from build123d import *

# Parameters (mm, degrees)
SKETCH_1_W      = 15
SKETCH_1_H      = 11
SKETCH_1_R      = 1.5
EXTRUDE_1_DEPTH = 1.5
SKETCH_2_W      = 5
SKETCH_2_H      = 5
EXTRUDE_2_DEPTH = 1


with BuildPart() as part:
    # 草图1 → 凸台-拉伸1 (new body)
    with BuildSketch(Plane.XY):
        Rectangle(SKETCH_1_W, SKETCH_1_H)
        with Locations((-5.5, 3.5)):
            Circle(SKETCH_1_R, mode=Mode.SUBTRACT)
        with Locations((5.5, 3.5)):
            Circle(SKETCH_1_R, mode=Mode.SUBTRACT)
    extrude(amount=EXTRUDE_1_DEPTH)

    # 草图2 → 凸台-拉伸2 (add)
    with BuildSketch(Plane.XY.offset(1.5)):
        Rectangle(SKETCH_2_W, SKETCH_2_H)
    extrude(amount=EXTRUDE_2_DEPTH)


solid = part.part
Check sheet for the modelled part. Datum: model origin and axes. Units: mm. A direction names the side the tool comes from. Give positions to 0.01 mm unless a question says otherwise; leave off trailing zeros. Loops run counter-clockwise (first coordinate to the right, second up) from the corner with the lowest first, then second, coordinate; pieces in that order, holes last. Notation, with made-up numbers: M 80.5,-21.75 L 85.5,-21.75 A22 ccw 85.5,-7.75 Z; hole C -36,-14.75 d5. An arc over 180 degrees is marked long. Return JSON: item names as keys, results as strings. Group by question number.
1. Cross-section at D-D on x = 1.25. Record the boundary of the cut face in (y, z).
2. Thickness scan on L1, parallel to Y at x = 5.5, z = 0.7; L2, parallel to Y at x = 1.5, z = 1.95; L3, parallel to X at y = 4.5, z = 0.2. Record the ranges inside material, lowest first.
3. Cross-section at C-C on y = -2.25. Record the boundary of the cut face in (x, z), plus the area to 3 significant figures.
4. Cross-section at A-A on y = 3.5. Record the boundary of the cut face in (x, z), plus the area to 3 significant figures.
5. Mould release check, pull along Y, two halves, no side actions. Record for faces 6 (the cylindrical face through (-7, 3.57, 0.74)), 7 (the flat face through (0, 0, 0)), 8 (the flat face through (0, -5.5, 1)), 9 (the flat face through (0, 5.5, 1)): released by +Y, released by -Y, zero draft, split by the parting line, or undercut.
6. Tool access check on faces 1 (the flat face through (2.5, 0, 2)), 2 (the flat face through (0, 2.5, 2)), 3 (the flat face through (-2.5, 0, 2)), 4 (the flat face through (0, -2.5, 2)), 5 (the flat face through (-7.5, 0, 1)). Record the directions out of +Z, -Z, +X, -X, +Y, -Y that give a thin tool (end or side, any length) a straight path to the whole face; none if there is none.
7. Go/stop test with flat-tipped pins: pin 1 (2.5 mm diameter, centred on x = -5.5, y = 3.5, fed in from -Z); pin 2 (0.5 mm diameter, centred on x = 0.5, z = 2, fed in from -Y); pin 3 (3.5 mm diameter, centred on x = 5.5, y = 3.5, fed in from +Z). Record where each tip stops, or that it passes through.
8. Cross-section at B-B on x = 5.5. Record the boundary of the cut face in (y, z), plus the area to 3 significant figures.
Return value:
{
 "1": {"outline": "M -5.5,0 L 5.5,0 L 5.5,1.5 L 2.5,1.5 L 2.5,2.5 L -2.5,2.5 L -2.5,1.5 L -5.5,1.5 Z"},
 "2": {"L1": "-5.5 to 2, 5 to 5.5", "L2": "-2.5 to 2.5", "L3": "-7.5 to -6.62, -4.38 to 4.38, 6.62 to 7.5"},
 "3": {"outline": "M -7.5,0 L 7.5,0 L 7.5,1.5 L 2.5,1.5 L 2.5,2.5 L -2.5,2.5 L -2.5,1.5 L -7.5,1.5 Z", "area": "27.5 mm^2"},
 "4": {"outline": "M -7.5,0 L -7,0 L -7,1.5 L -7.5,1.5 Z; M -4,0 L 4,0 L 4,1.5 L -4,1.5 Z; M 7,0 L 7.5,0 L 7.5,1.5 L 7,1.5 Z", "area": "13.5 mm^2"},
 "5": {"face 6": "undercut", "face 7": "zero draft", "face 8": "released by -Y", "face 9": "released by +Y"},
 "6": {"face 1": "+Z, +X, +Y, -Y", "face 2": "+Z, +X, -X, +Y", "face 3": "+Z, -X, +Y, -Y", "face 4": "+Z, +X, -X, -Y", "face 5": "+Z, -Z, -X, +Y, -Y"},
 "7": {"pin 1": "through", "pin 2": "y = -2.5", "pin 3": "z = 1.5"},
 "8": {"outline": "M -5.5,0 L 2,0 L 2,1.5 L -5.5,1.5 Z; M 5,0 L 5.5,0 L 5.5,1.5 L 5,1.5 Z", "area": "12.0 mm^2"}
}
